Can you work these out from the model? Positions are in its coordinate system, mm. A direction names the side the tool comes from. Coordinates: 2 decimals unless noted, no trailing zeros. Loops run counter-clockwise (first coordinate to the right, second up) from the corner with the lowest first, then second, coordinate; pieces in that order, holes last.
```python
from build123d import *

# Parameters (mm, degrees)
SM_BASE_FLANGE_1_DEPTH = 233


# Sheet-metal steps are written as plain solids
with BuildPart() as part:
    # 草图1 → 基体-法兰1 (new body)
    with BuildSketch(Plane(origin=(0, 0, 0), x_dir=(1, 0, 0), z_dir=(0, 1, 0))):
        with BuildLine():
            Line((-129, 230), (-172.917182347, 192.646402715))
            ThreePointArc((-172.917182347, 192.646402715), (-173.157776183, 192.403386175), (-173.353453197, 192.122934861))
            Line((-173.353453197, 192.122934861), (-249.622758888, 60.020622347))
            ThreePointArc((-249.622758888, 60.020622347), (-249.864241735, 59.344913751), (-249.8516834, 58.627461063))
            Line((-249.8516834, 58.627461063), (-240.235572229, 10.665066397))
            ThreePointArc((-240.235572229, 10.665066397), (-240.145872891, 10.352305448), (-240.006647716, 10.058227681))
            Line((-240.006647716, 10.058227681), (-106.206165205, -221.691006107))
            ThreePointArc((-106.206165205, -221.691006107), (-106.021098975, -221.958617528), (-105.795089717, -222.192679908))
            Line((-105.795089717, -222.192679908), (-69.066493095, -254.501673801))
            ThreePointArc((-69.066493095, -254.501673801), (-68.451440008, -254.871275982), (-67.745517775, -255))
            Line((-67.745517775, -255), (67.745517775, -255))
            ThreePointArc((67.745517775, -255), (68.451440008, -254.871275982), (69.066493095, -254.501673801))
            Line((69.066493095, -254.501673801), (105.795089717, -222.192679908))
            ThreePointArc((105.795089717, -222.192679908), (106.021098975, -221.958617528), (106.206165205, -221.691006107))
            Line((106.206165205, -221.691006107), (240.006647716, 10.058227681))
            ThreePointArc((240.006647716, 10.058227681), (240.145872891, 10.352305448), (240.235572229, 10.665066397))
            Line((240.235572229, 10.665066397), (249.8516834, 58.627461063))
            ThreePointArc((249.8516834, 58.627461063), (249.864241735, 59.344913751), (249.622758888, 60.020622347))
            Line((249.622758888, 60.020622347), (173.353453197, 192.122934861))
            ThreePointArc((173.353453197, 192.122934861), (173.157776183, 192.403386175), (172.917182347, 192.646402715))
            Line((172.917182347, 192.646402715), (129, 230))
            Line((129, 230), (129.647889979, 230.761733927))
            Line((129.647889979, 230.761733927), (173.565072326, 193.408136642))
            ThreePointArc((173.565072326, 193.408136642), (173.92596308, 193.043611831), (174.219478601, 192.622934861))
            Line((174.219478601, 192.622934861), (250.488784291, 60.520622347))
            ThreePointArc((250.488784291, 60.520622347), (250.851008562, 59.507059453), (250.83217106, 58.430880421))
            Line((250.83217106, 58.430880421), (241.216059889, 10.468485755))
            ThreePointArc((241.216059889, 10.468485755), (241.081510882, 9.999344331), (240.87267312, 9.558227681))
            Line((240.87267312, 9.558227681), (107.072190608, -222.191006107))
            ThreePointArc((107.072190608, -222.191006107), (106.794591264, -222.592423239), (106.455577377, -222.943516809))
            Line((106.455577377, -222.943516809), (69.726980755, -255.252510702))
            ThreePointArc((69.726980755, -255.252510702), (68.804401125, -255.806913973), (67.745517775, -256))
            Line((67.745517775, -256), (-67.745517775, -256))
            ThreePointArc((-67.745517775, -256), (-68.804401125, -255.806913973), (-69.726980755, -255.252510702))
            Line((-69.726980755, -255.252510702), (-106.455577377, -222.943516809))
            ThreePointArc((-106.455577377, -222.943516809), (-106.794591264, -222.592423239), (-107.072190608, -222.191006107))
            Line((-107.072190608, -222.191006107), (-240.87267312, 9.558227681))
            ThreePointArc((-240.87267312, 9.558227681), (-241.081510882, 9.999344331), (-241.216059889, 10.468485754))
            Line((-241.216059889, 10.468485755), (-250.83217106, 58.430880421))
            ThreePointArc((-250.83217106, 58.430880421), (-250.851008562, 59.507059453), (-250.488784291, 60.520622347))
            Line((-250.488784291, 60.520622347), (-174.219478601, 192.622934861))
            ThreePointArc((-174.219478601, 192.622934861), (-173.92596308, 193.043611831), (-173.565072326, 193.408136642))
            Line((-173.565072326, 193.408136642), (-129.647889979, 230.761733927))
            Line((-129.647889979, 230.761733927), (-129, 230))
        make_face()
    extrude(amount=SM_BASE_FLANGE_1_DEPTH)


solid = part.part
```
Item 1: I need wall thicknesses on line 1 along Z through (x, y) = (-59, 201); line 2 along X through (y, z) = (53, -111.5); line 3 along X through (y, z) = (160.5, -45). Which ranges of each line are inside material? Lowest first, please.
Results are:
line 1: z = 255 to 256
line 2: x = -221.06 to -219.9, 219.9 to 221.06
line 3: x = -248.14 to -247.12, 247.12 to 248.14
Item 2: On a 3-axis mill with a long thin cutter (end or side, diameter ignored), from which of +Z, -Z, +X, -X, +Y, -Y can I reach the whole of each face in a straight line? I mean faces 5 (the face through (-87.69, 114.87, 238.12)), 6 (the face through (151.299, 114.869, -212.346)), 7 (the face through (-245.11, 114.87, -34.98)). Say none if no direction works.
Results are:
face 5: -Z, +Y, -Y
face 6: -Z, +X, +Y, -Y
face 7: +Y, -Y
Item 3: Suppose I cut it at B-B, the plane z = -159. Please give me the cut outline in (x, y).
Results are:
outline: (-193.63, 0) - (-192.48, 0) - (-192.48, 233) - (-193.63, 233) - close; (192.48, 0) - (193.63, 0) - (193.63, 233) - (192.48, 233) - close
Item 4: Suppose I cut it at A-A, the plane x = -145.5. Please give me the cut outline in (y, z), plus the area to 3 significant figures.
Results are:
outline: (0, -217.28) - (233, -217.28) - (233, -215.97) - (0, -215.97) - close; (0, 153.63) - (233, 153.63) - (233, 155.63) - (0, 155.63) - close
area: 772 mm2
Item 5: I'm going to push flat-ended pins straight in: P1, Ø1.5, axis at y = 35, z = 87.5, coming from the -X side; P2, Ø12, axis at y = 199, z = -154.5, coming from the +X side; P3, Ø8, axis at y = 121, z = 147, coming from the +X side. Where does each tip first touch, or does it pass through?
Results are:
P1: stops at x = -185.27
P2: stops at x = 199.69
P3: stops at x = 152.79
Item 6: We'd pull the mould along Z, two halves only. Please class faces 1 (the face through (-173, 115, 108)), 2 (the face through (-1, 115, 255)), 3 (the face through (244.976, 114.869, -34.311)), 4 (the face through (172.17, 114.87, 107.44)): +Z half, -Z half, draft (parallel to the pull), parting line (faces both ways), or undercut.
Results are:
face 1: +Z half
face 2: -Z half
face 3: undercut
face 4: undercut
Item 7: Suppose I cut it at C-C, the plane x = 47. Please give me the cut outline in (y, z), plus the area to 3 significant figures.
Results are:
outline: (0, 255) - (233, 255) - (233, 256) - (0, 256) - close
area: 233 mm2
